The listing builds one solid part. Answer for the finished solid, in the listing's coordinates (mm). A direction names the side the tool comes from. Coordinates: 2 decimals unless noted, no trailing zeros. Order: outer loops, then holes, each group sorted by start corner. A loop starts at its lowest first (then second) coordinate and runs counter-clockwise, first axis right, second up. Notation, with made-up numbers: (-10.5, 5.5) - (36.5, 5.5) arc R18 cw to (36.5, 13.5) - close; hole circle Ø7 at (42, 35.25). An arc over 180 degrees is marked (long way). Use a Markdown table: item, result. Add a question column.
Item 1: Find the intervals of material crossed by line 1 along X through (y, z) = (-9, 2.75); line 2 along Z through (x, y) = (5, -16.5), in increasing order.
Item 2: Flat-ended cylindrical pins translate along their axes: P1, Ø6, axis at x = 6, y = -24, coming from the +Z side; P2, Ø4, axis at x = 23, y = -26, coming from the -Z side. Find the tip coordinate at first contact, or state that the pin passes through.
Item 3: The part is cut by section C-C, the plane x = 16.5. Give the vertices of the cut face in (y, z), then the cut area to 3 significant figures.
Item 4: For faces 5 (the flat face through (0, -19, 8)), 6 (the flat face through (-1, -18, 14)), 7 (the flat face through (-1, -7, 8)), determine the directions among +Z, -Z, +X, -X, +Y, -Y from which every point of the face is accessible in a straight line to the end or side of a thin tool.
Item 5: The part is cut by section D-D, the plane y = -6. Give the vertices of the cut face in (x, z), then the cut area to 3 significant figures.
Item 6: The part is cut by section A-A, the plane z = 5.5. Give the vertices of the cut face in (x, y), then the cut area to 3 significant figures.
Item 7: The part is cut by section B-B, the plane y = -18.5. Give the vertices of the cut face in (x, z), then the cut area to 3 significant figures.
Item 8: The mould has two halves that part along Y. Classify faces 1 (the flat face through (12.4, 0, 1.8)), 2 (the flat face through (26, -4.5, 8)), 3 (the flat face through (12, -15, 0)), 4 (the flat face through (12.4, -30, 1.8)): released by +Y, released by -Y, zero draft, split by the parting line, or undercut.
from build123d import *

# Parameters (mm, degrees)
F0_W     = 2
F0_H     = 2.5
F1_DEPTH = 2
F0_H_2   = 23
F0_H_3   = 4.5
F2_DEPTH = 14


with BuildPart() as f1:
    # F0 (on Top) → F1 (new body)
    with BuildSketch(Plane.XY):
        Polygon((12.5, 0), (0, 0), (0, -4.5), (0, -7), (0, -30), (12.5, -30), align=None)
        Polygon((25, 0), (12.5, 0), (12.5, -30), (25, -30), (25, -7), (25, -4.5), align=None)
        with Locations((-1, -5.75)):
            Rectangle(F0_W, F0_H)
        with Locations((26, -5.75)):
            Rectangle(F0_W, F0_H)
    extrude(amount=F1_DEPTH)

    # F0 (on Top) → F2 (join)
    with BuildSketch(Plane.XY):
        with Locations((-1, -18.5)):
            Rectangle(F0_W, F0_H_2)
        with Locations((-1, -2.25)):
            Rectangle(F0_W, F0_H_3)
        with Locations((26, -2.25)):
            Rectangle(F0_W, F0_H_3)
        with Locations((26, -18.5)):
            Rectangle(F0_W, F0_H_2)
    extrude(amount=F2_DEPTH)


solid = f1.part
Solution:
| question | item | result |
|---|---|---|
| 1 | line 1 | x = -2 to 0, 25 to 27 |
| 1 | line 2 | z = 0 to 2 |
| 2 | P1 | stops at z = 2 |
| 2 | P2 | stops at z = 0 |
| 3 | outline | (-30, 0) - (0, 0) - (0, 2) - (-30, 2) - close |
| 3 | area | 60.0 mm2 |
| 4 | face 5 | +Z, +Y, -Y |
| 4 | face 6 | +Z, +X, -X, +Y, -Y |
| 4 | face 7 | +Z, +X, -X |
| 5 | outline | (-2, 0) - (27, 0) - (27, 2) - (-2, 2) - close |
| 5 | area | 58.0 mm2 |
| 6 | outline | (-2, -30) - (0, -30) - (0, -7) - (-2, -7) - close; (-2, -4.5) - (0, -4.5) - (0, 0) - (-2, 0) - close; (25, -30) - (27, -30) - (27, -7) - (25, -7) - close; (25, -4.5) - (27, -4.5) - (27, 0) - (25, 0) - close |
| 6 | area | 110 mm2 |
| 7 | outline | (-2, 0) - (27, 0) - (27, 14) - (25, 14) - (25, 2) - (0, 2) - (0, 14) - (-2, 14) - close |
| 7 | area | 106 mm2 |
| 8 | face 1 | released by +Y |
| 8 | face 2 | undercut |
| 8 | face 3 | zero draft |
| 8 | face 4 | released by -Y |
